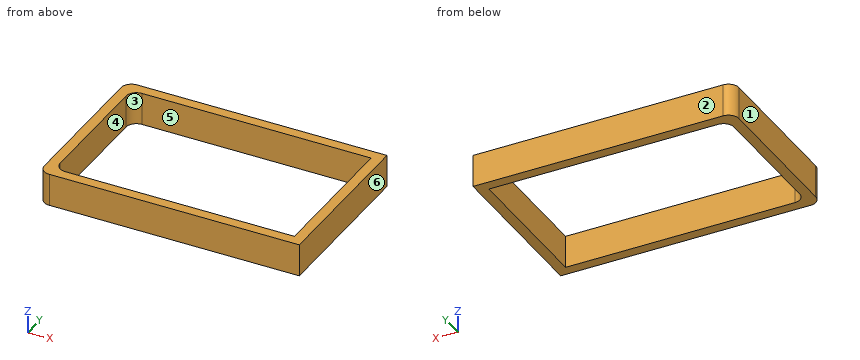
from build123d import *

# Parameters (mm, degrees)
F1_DEPTH = 19.812


with BuildPart() as f1:
    # F0 (on Top) → F1 (new body)
    with BuildSketch(Plane.XY):
        with BuildLine():
            Line((105.372425, 55.590845), (-47.027575, 55.590845))
            ThreePointArc((-47.027575, 55.590845), (-51.517703, 53.730973), (-53.377575, 49.240845))
            Line((-53.377575, 49.240845), (-53.377575, -39.659155))
            ThreePointArc((-53.377575, -39.659155), (-51.517703, -44.149283), (-47.027575, -46.009155))
            Line((-47.027575, -46.009155), (105.372425, -46.009155))
            Line((105.372425, -46.009155), (105.372425, 55.590845))
        make_face()
        Polygon((-47.027575, 42.890845), (-47.027575, 49.240845), (-40.677575, 49.240845), (99.022425, 49.240845), (99.022425, -39.659155), (-40.677575, -39.659155), (-47.027575, -39.659155), (-47.027575, -33.309155), align=None, mode=Mode.SUBTRACT)
        with BuildLine():
            Line((-40.677575, 49.240845), (-47.027575, 49.240845))
            Line((-47.027575, 49.240845), (-47.027575, 42.890845))
            ThreePointArc((-47.027575, 42.890845), (-45.167703, 47.380973), (-40.677575, 49.240845))
        make_face()
        with BuildLine():
            ThreePointArc((-40.677575, -39.659155), (-45.167703, -37.799283), (-47.027575, -33.309155))
            Line((-47.027575, -33.309155), (-47.027575, -39.659155))
            Line((-47.027575, -39.659155), (-40.677575, -39.659155))
        make_face()
    extrude(amount=F1_DEPTH)


solid = f1.part
Could you check a few things on this model? Use its own coordinates, in mm. Face numbers are marked on the shaded views. A direction names the side the tool comes from. Coordinates: 2 decimals unless noted, no trailing zeros. Loops run counter-clockwise (first coordinate to the right, second up) from the corner with the lowest first, then second, coordinate; pieces in that order, holes last.
1. Imagine slicing it at A-A (y = -24). Please give me the cut outline in (x, z), and give its area (3 significant figures).
2. I need wall thicknesses on L1, parallel to Y at x = -3, z = 12.5; L2, parallel to X at y = 27, z = 13; L3, parallel to Y at x = -45, z = 8.25. Which ranges of each line are inside material? Lowest first, please.
3. Imagine slicing it at C-C (z = 17.25). Please give me the cut outline in (x, y).
4. For the marked faces 5 and 6, which set-ups out of +Z, -Z, +X, -X, +Y, -Y let a thin tool reach every point of the face, with its end or its side?
5. We'd pull the mould along Y, two halves only. Please class the marked faces 1, 2, 3 and 4: released by +Y, released by -Y, zero draft, split by the parting line, or undercut.
6. Imagine slicing it at B-B (x = 83). Please give me the cut outline in (y, z), and give its area (3 significant figures).
Computed values:
1. outline: (-53.38, 0) - (-47.03, 0) - (-47.03, 19.81) - (-53.38, 19.81) - close; (99.02, 0) - (105.37, 0) - (105.37, 19.81) - (99.02, 19.81) - close
1. area: 252 mm2
2. L1: y = -46.01 to -39.66, 49.24 to 55.59
2. L2: x = -53.38 to -47.03, 99.02 to 105.37
2. L3: y = -46.01 to -37.96, 47.54 to 55.59
3. outline: (-53.38, -39.66) arc R6.35 ccw to (-47.03, -46.01) - (105.37, -46.01) - (105.37, 55.59) - (-47.03, 55.59) arc R6.35 ccw to (-53.38, 49.24) - close; hole (-47.03, -33.31) arc R6.35 ccw to (-40.68, -39.66) - (99.02, -39.66) - (99.02, 49.24) - (-40.68, 49.24) arc R6.35 ccw to (-47.03, 42.89) - close
4. face 5: +Z, -Z
4. face 6: +Z, -Z, +X, +Y, -Y
5. face 1: zero draft
5. face 2: released by +Y
5. face 3: undercut
5. face 4: undercut
6. outline: (-46.01, 0) - (-39.66, 0) - (-39.66, 19.81) - (-46.01, 19.81) - close; (49.24, 0) - (55.59, 0) - (55.59, 19.81) - (49.24, 19.81) - close
6. area: 252 mm2
